Here's the drawing with two shaded views (mm, measured from the low corner). I have some questions. A direction names the side the tool comes from. Give positions to 0.01 mm unless a question says otherwise; leave off trailing zeros. Write each loop counter-clockwise with the first axis right and the second up, starting at its lowest first coordinate (ties: lowest second). Pieces come first, ordered by that corner, then holes.
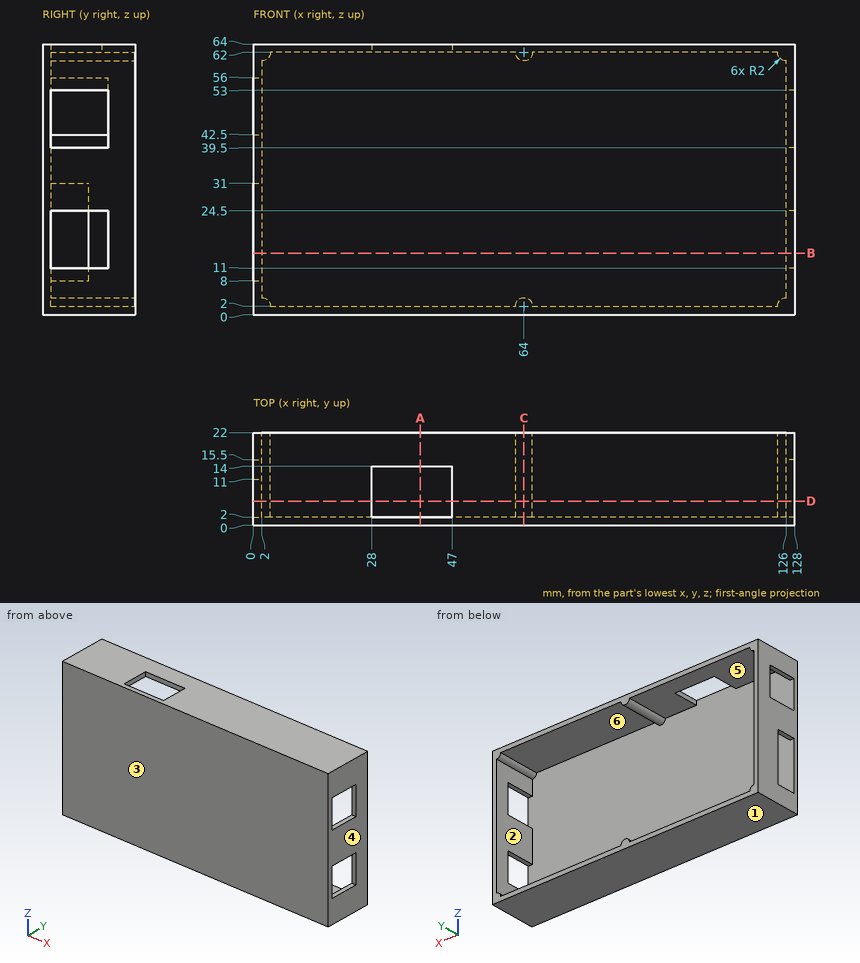
(1) Imagine slicing it at D-D, the plane y = 5.75. Give the number of separate pieces and of enclosed holes in the cut face, plus the area to 3 significant figures.
Returned:
separate pieces: 5
enclosed holes: 0
area: 612 mm2
(2) Imagine slicing it at B-B, the plane z = 14.5. Write out the boundary of the cut face in (x, y), plus the area to 3 significant figures.
Returned:
outline: (0, 0) - (128, 0) - (128, 2) - (0, 2) - close; (0, 11) - (2, 11) - (2, 22) - (0, 22) - close; (126, 15.5) - (128, 15.5) - (128, 22) - (126, 22) - close
area: 291 mm2
(3) If I drill on L1, parallel to Z at x = 75, y = 20.25; L2, parallel to X at y = 20.25, z = 54; L3, parallel to X at y = 4, z = 3.5, over which ranges is the centre line in solid material (lowest first)?
Returned:
L1: z = 0 to 2, 62 to 64
L2: x = 0 to 2, 126 to 128
L3: x = 0 to 3.32, 62.68 to 65.32, 124.68 to 128
(4) Imagine slicing it at A-A, the plane x = 39.5. Write out the boundary of the cut face in (y, z), plus the area to 3 significant figures.
Returned:
outline: (0, 0) - (22, 0) - (22, 2) - (2, 2) - (2, 64) - (0, 64) - close; (14, 62) - (22, 62) - (22, 64) - (14, 64) - close
area: 184 mm2
(5) Will this pin go through, and if not, where does the flat tip stop? P1, Ø18.5, axis at x = 79, z = 19, coming from the +Y side.
Returned:
P1: stops at y = 2
(6) For the marked faces 1 and 2, which set-ups out of +Z, -Z, +X, -X, +Y, -Y let a thin tool reach every point of the face, with its end or its side?
Returned:
face 1: -Z, +X, -X, +Y, -Y
face 2: +Y
(7) If we mould it in two halves opening along X, with no side actions, what happens to the marked faces 3, 4, 5 and 6? For each: +X half, -X half, draft (parallel to the pull), parting line (faces both ways), or undercut.
Returned:
face 3: draft
face 4: +X half
face 5: undercut
face 6: undercut
(8) Imagine slicing it at C-C, the plane x = 64. Write out the boundary of the cut face in (y, z), plus the area to 3 significant figures.
Returned:
outline: (0, 0) - (22, 0) - (22, 4) - (2, 4) - (2, 60) - (22, 60) - (22, 64) - (0, 64) - close
area: 288 mm2
